Design review of the part built by this model. Coordinates are the model's own, in mm. Face numbers are marked on the shaded views. A direction names the side the tool comes from. Coordinates: 2 decimals unless noted, no trailing zeros. Order: outer loops, then holes, each group sorted by start corner. A loop starts at its lowest first (then second) coordinate and runs counter-clockwise, first axis right, second up. Notation, with made-up numbers: M -6,66.25 L 22,66.25 A18 ccw 22,86.25 Z; hole C -27.75,-35 d6. An arc over 180 degrees is marked long. Answer in a Markdown table with one row per item.
from build123d import *

# Parameters (mm, degrees)
F1_DEPTH = 20
F2_R     = 8
F3_R     = 2.49999


# Not quite as in the source:
# - a fillet or chamfer is up to 0.001 mm smaller than in the source, because OpenCascade refuses the exact size


with BuildPart() as f1:
    # F0 (on Front) → F1 (new body)
    with BuildSketch(Plane.XZ):
        Polygon((-35, 0), (-29.5880389985, 0), (0, 71.4318450343), (0, 84.4974746831), align=None)
        Polygon((0, 71.4318450343), (29.5880389985, 0), (35, 0), (0, 84.4974746831), align=None)
        Polygon((0, -5), (0, 0), (-29.5880389985, 0), (-35, 0), (-60, 0), (-67.0710678119, 7.0710678119), (-71.5539451727, 4.4828773608), (-63.5355339059, -3.5355339059), (-60, -5), align=None)
        Polygon((29.5880389985, 0), (0, 0), (0, -5), (60, -5), (63.5355339059, -3.5355339059), (71.5539451727, 4.4828773608), (67.0710678119, 7.0710678119), (60, 0), (35, 0), align=None)
    extrude(amount=F1_DEPTH)

    # F2
    f2_edges = [f1.edges().sort_by_distance(p)[0] for p in [
        (0, -10, 84.497475),
        (0, -10, 71.431845),
    ]]
    fillet(f2_edges, radius=F2_R)

    # F3 (radius 2.5 in the source; OpenCascade refuses exactly that, so slightly less here)
    f3_edges = [f1.edges().sort_by_distance(p)[0] for p in [
        (-67.071068, -10, 7.071068),
        (-71.553945, -10, 4.482877),
        (67.071068, -10, 7.071068),
        (71.553945, -10, 4.482877),
    ]]
    fillet(f3_edges, radius=F3_R)


solid = f1.part
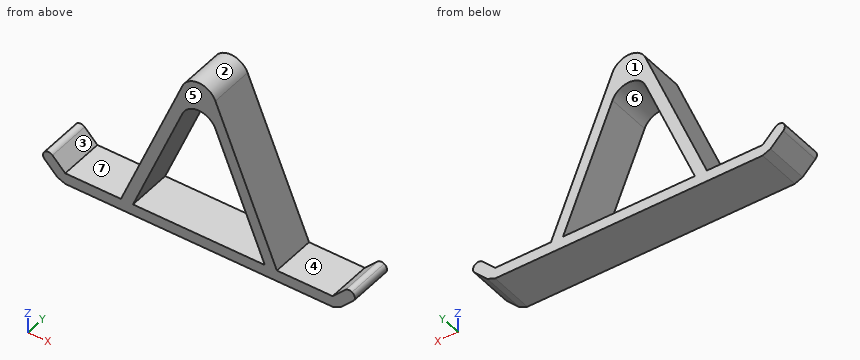
(1) Add section B-B, the plane x = -2. Give the boundary of the cut face in (y, z), and give its area (3 significant figures).
Return value:
| item | result |
|---|---|
| outline | M -20,-5 L 0,-5 L 0,0 L -20,0 Z; M -20,58.27 L 0,58.27 L 0,71.34 L -20,71.34 Z |
| area | 361 mm2 |
(2) For line 1 along Z through (x, y) = (-35.5, -14.75); line 2 along Z through (x, y) = (14, -5.75); line 3 along X through (y, z) = (-8.75, 27.5), list the stretches that pass through material, from the lowest coordinate up. Write a range as from..to.
Return value:
| item | result |
|---|---|
| line 1 | z = -5..0 |
| line 2 | z = -5..0, 37.63..50.7 |
| line 3 | x = -23.61..-18.2, 18.2..23.61 |
(3) For the marked faces 5, 6 and 7, list the 3-axis set-ups (+Z, -Z, +X, -X, +Y, -Y) from which the entire face can be reached by the end or side of a thin tool; tool diameter is ignored.
Return value:
| item | result |
|---|---|
| face 5 | +Z, -Z, +X, -X, -Y |
| face 6 | +Y, -Y |
| face 7 | +Z, +Y, -Y |
(4) Add section D-D, the plane z = 23.5. Give the boundary of the cut face in (x, y), and give its area (3 significant figures).
Return value:
| item | result |
|---|---|
| outline | M -25.27,-20 L -19.85,-20 L -19.85,0 L -25.27,0 Z; M 19.85,-20 L 25.27,-20 L 25.27,0 L 19.85,0 Z |
| area | 216 mm2 |
(5) Insertion check: pin 1 Ø10 at (x, y) = (-34.5, -15) entering from +Z; pin 2 Ø10 at (y, z) = (-5, 34.5) entering from -X; pin 3 Ø4 at (y, z) = (-10.5, 40) entering from -X. Each pin has a flat end and moves straight along its axis. Give the tip position at first contact, or say it passes through.
Return value:
| item | result |
|---|---|
| pin 1 | stops at z = 13.28 |
| pin 2 | stops at x = -22.78 |
| pin 3 | stops at x = -19.26 |
(6) Add section C-C, the plane z = 4. Give the boundary of the cut face in (x, y), and give its area (3 significant figures).
Return value:
| item | result |
|---|---|
| outline | M -69.98,-20 L -64,-20 L -64,0 L -69.98,0 Z; M -33.34,-20 L -27.93,-20 L -27.93,0 L -33.34,0 Z; M 27.93,-20 L 33.34,-20 L 33.34,0 L 27.93,0 Z; M 64,-20 L 69.98,-20 L 69.98,0 L 64,0 Z |
| area | 456 mm2 |
(7) Draft analysis for pull direction X (two halves, no side actions). For the marked faces 1, 2, 3 and 4, state which applies: pulls with the +X half, pulls with the -X half, needs draft (parallel to the pull), parting line crosses it, or undercut.
Return value:
| item | result |
|---|---|
| face 1 | needs draft |
| face 2 | parting line crosses it |
| face 3 | undercut |
| face 4 | undercut |
